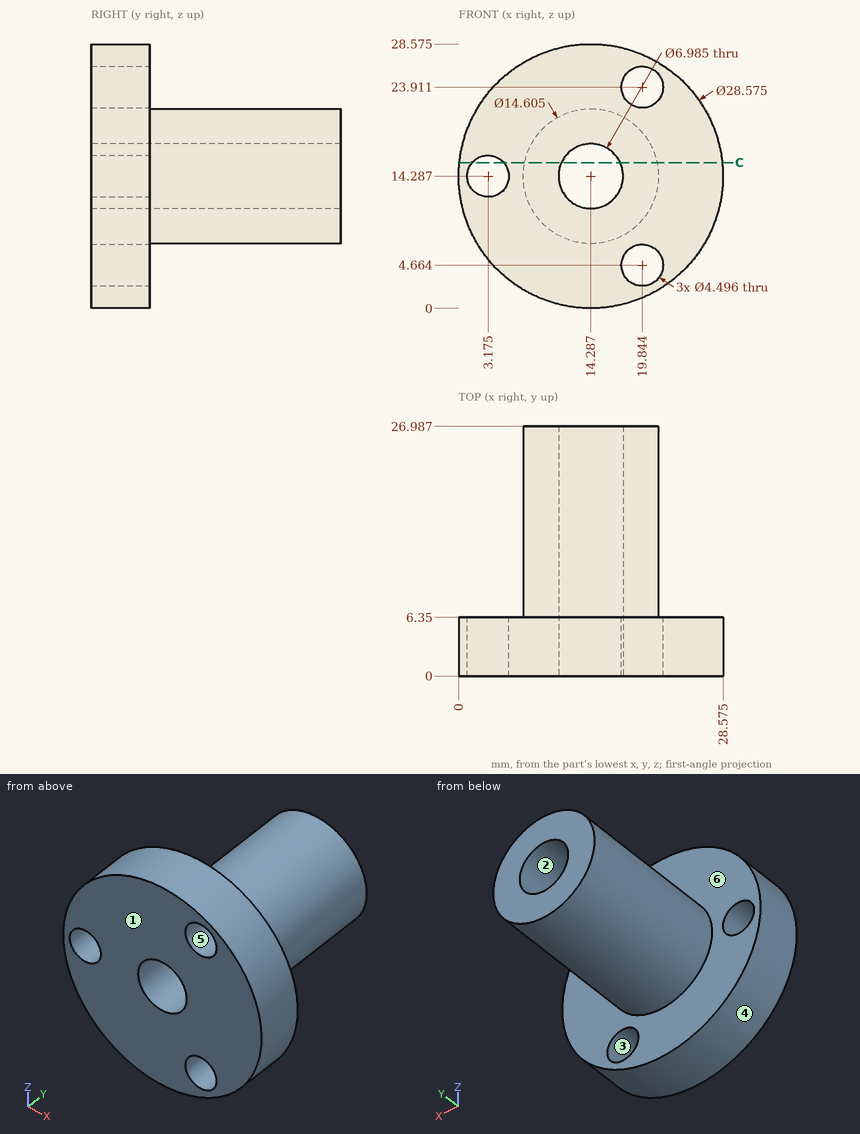
Source: three-view drawing plus pictorial views. Frame: mm from the lowest corner of the part. A direction names the side the tool comes from. Coordinates: 2 decimals unless noted, no trailing zeros.
Item 1: Cut plane C-C (z = 15.75). Count the separate pieces of the cut face and the enclosed holes in it, plus the area to 3 significant figures.
Output values:
separate pieces: 3
enclosed holes: 0
area: 283 mm2
Item 2: Material intervals for line 1 (Y direction, x = 5, z = 16.25); line 2 (X direction, y = 5.5, z = 23) (1 decimal); line 3 (X direction, y = 13.25, z = 20) (1 decimal), sorted ascending.
Output values:
line 1: y = 0 to 6.35
line 2: x = 3 to 17.8, 21.9 to 25.6
line 3: x = 9.7 to 18.8
Item 3: Set-up query: the marked faces 5 and 6. Return all of +Z, -Z, +X, -X, +Y, -Y with unobstructed straight access to the full face (end or side cutting, diameter ignored); none if empty.
Output values:
face 5: +Y, -Y
face 6: +Y
Item 4: First-contact query: P1, Ø3, axis at x = 5, y = 7, coming from the -Z side (1 decimal); P2, Ø1, axis at x = 17, y = 7, coming from the -Z side; P3, Ø1, axis at y = 18, z = 8.5, coming from the -X side. Flat tips, straight axial feed; report the tip coordinate or a pass-through.
Output values:
P1: stops at z = 2.4
P2: stops at z = 7.33
P3: stops at x = 9.25
Item 5: Pull-direction query (Z, two-part tool) for the marked faces 1, 2, 3 and 4; classes: pulls with the +Z half, pulls with the -Z half, needs draft (parallel to the pull), parting line crosses it, or undercut.
Output values:
face 1: needs draft
face 2: undercut
face 3: undercut
face 4: parting line crosses it
